Job drawing, mm, ordinate dimensions from the low corner. One solid piece. A direction names the side the tool comes from. Give positions to 0.01 mm unless a question says otherwise; leave off trailing zeros. Loops run counter-clockwise (first coordinate to the right, second up) from the corner with the lowest first, then second, coordinate; pieces in that order, holes last.
Item 1: Saw through at C-C on z = 4.5. Give the cut face in (x, y) (3 decimals).
Item 2: Drop a flat-ended pin along its axis: P1, Ø1.5, axis at y = 1.5, z = 2, coming from the +X side (3 decimals). Give the stop position or say it passes through.
Item 3: Saw through at A-A on y = 1.75. Give the cut face in (x, z) (3 decimals), plus the area to 3 significant figures.
Item 4: Mould opens along Z. For the marked faces 3, 4 and 5 say: released by +Z, released by -Z, zero draft, split by the parting line, or undercut.
Item 5: Probe probe 1 along Z at (x, y) = (0.5, 1.5); probe 2 along Y at (x, z) = (2, 6.75); probe 3 along Y at (x, z) = (2.8, 0.75). List the from-to ranges inside material, lowest first.
Item 6: Which spindle directions (+Z, -Z, +X, -X, +Y, -Y) get a long thin tool onto all of the face, cutting with end or side? Do the marked faces 1 and 2. Say none if no direction does.
Item 7: Saw through at D-D on x = 0.7. Give the cut face in (y, z).
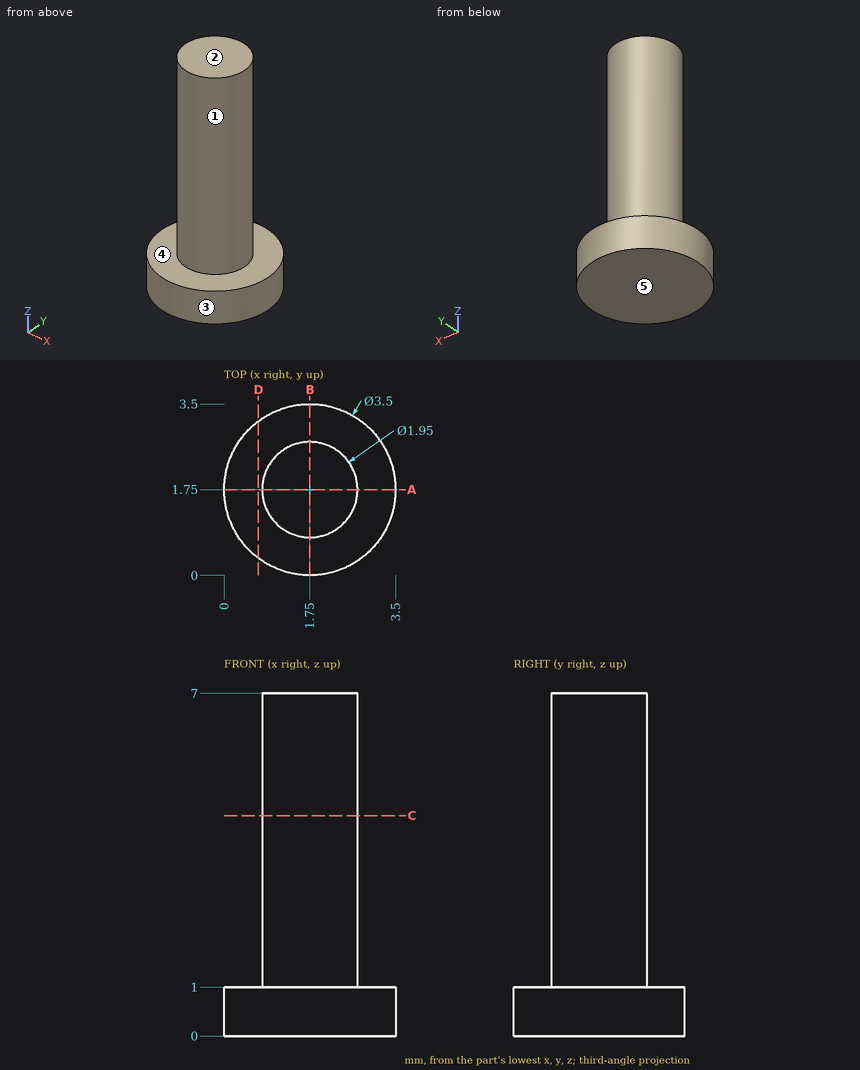
Results below:
1. outline: circle Ø1.95 at (1.75, 1.75)
2. P1: stops at x = 2.725
3. outline: (0, 0) - (3.5, 0) - (3.5, 1) - (2.725, 1) - (2.725, 7) - (0.775, 7) - (0.775, 1) - (0, 1) - close
3. area: 15.2 mm2
4. face 3: zero draft
4. face 4: released by +Z
4. face 5: released by -Z
5. probe 1: z = 0 to 1
5. probe 2: y = 0.81 to 2.69
5. probe 3: y = 0.35 to 3.15
6. face 1: +Z
6. face 2: +Z, +X, -X, +Y, -Y
7. outline: (0.35, 0) - (3.15, 0) - (3.15, 1) - (0.35, 1) - close
